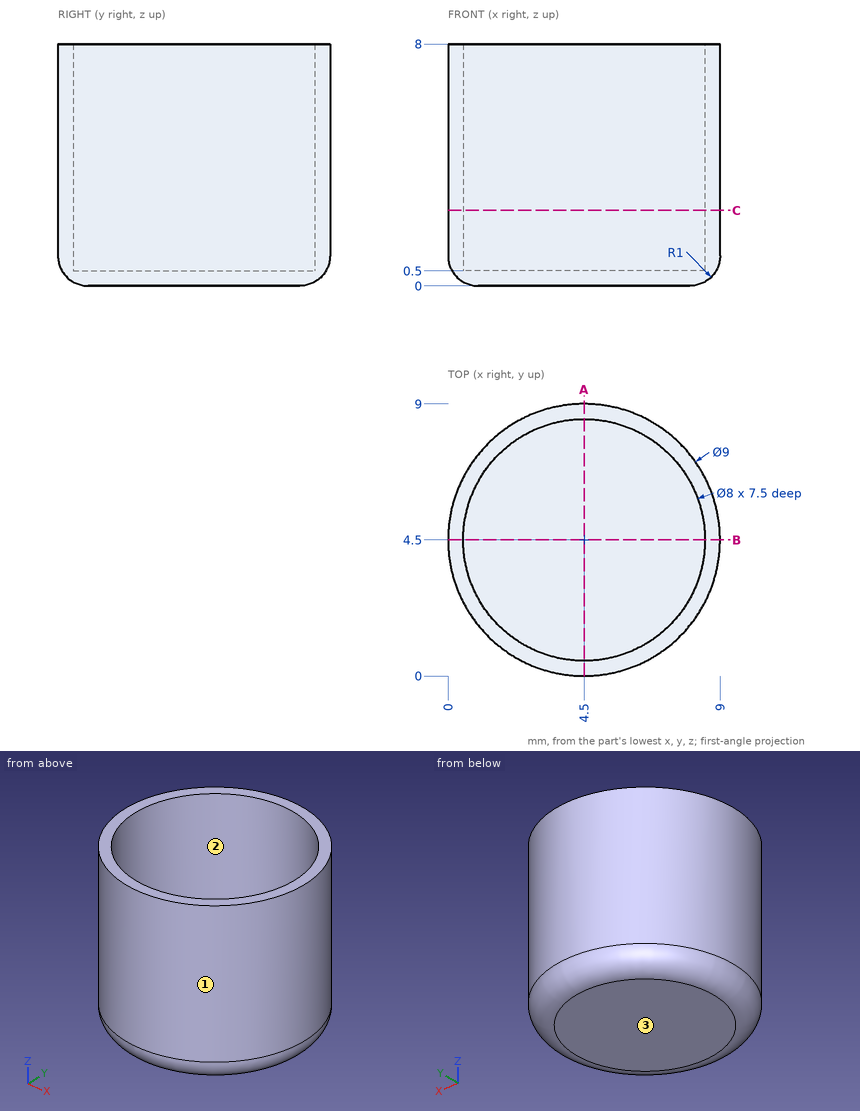
Here's the drawing with two shaded views (mm, measured from the low corner). I have some questions. Coordinates: 2 decimals unless noted, no trailing zeros. Loops run counter-clockwise (first coordinate to the right, second up) from the corner with the lowest first, then second, coordinate; pieces in that order, holes last. Notation, with made-up numbers: M -26,47 L 32,47 A11 cw 32,51 Z; hole C 80.25,-28.5 d9. An arc over 180 degrees is marked long. Put each result on its own line as item: value. Start each with the question number.
(1) Imagine slicing it at A-A on x = 4.5. List the corners of the cut face in (y, z) for me.
(2) Will these pins go through, and if not, where does the flat tip stop? pin 1 Ø2 at (x, z) = (3, 5.5) entering from -Y; pin 2 Ø1.5 at (x, z) = (8, 7) entering from +Y.
(3) Imagine slicing it at C-C on z = 2.5. List the corners of the cut face in (x, y) for me, and give its area (3 significant figures).
(4) We'd pull the mould along Y, two halves only. Please class the marked faces 1, 2 and 3: +Y half, -Y half, draft (parallel to the pull), parting line (faces both ways), or undercut.
(5) I need wall thicknesses on probe 1 along Y at (x, z) = (4.5, 2); probe 2 along Y at (x, z) = (7.5, 7); probe 3 along X at (y, z) = (6.5, 4.5). Which ranges of each line are inside material? Lowest first, please.
Worked answers:
1. outline: M 0,1 A1 ccw 1,0 L 8,0 A1 ccw 9,1 L 9,8 L 8.5,8 L 8.5,0.5 L 0.5,0.5 L 0.5,8 L 0,8 Z
2. pin 1: stops at y = 0.03
2. pin 2: stops at y = 8.06
3. outline: C 4.5,4.5 d9; hole C 4.5,4.5 d8
3. area: 13.4 mm2
4. face 1: parting line
4. face 2: undercut
4. face 3: draft
5. probe 1: y = 0 to 0.5, 8.5 to 9
5. probe 2: y = 1.15 to 1.85, 7.15 to 7.85
5. probe 3: x = 0.47 to 1.04, 7.96 to 8.53
